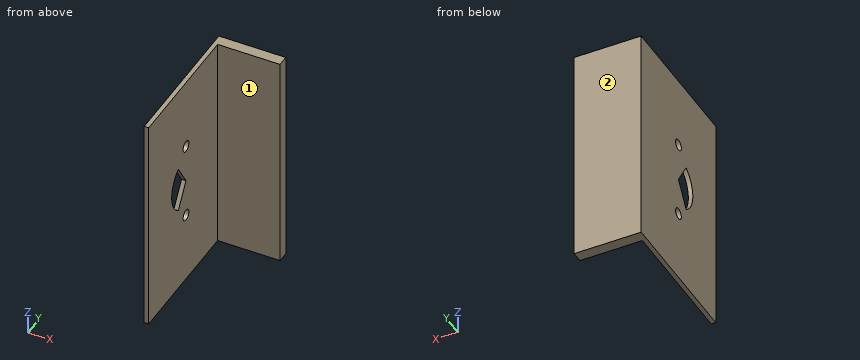
```python
from build123d import *

# Parameters (mm, degrees)
SKETCH1_W           = 100
SKETCH1_H           = 5
BOSS_EXTRUDE5_DEPTH = 2
SKETCH4_W           = 100
SKETCH4_H           = 5
BOSS_EXTRUDE6_DEPTH = 28


with BuildPart() as part:
    # Sketch1 → Boss-Extrude5 (new body)
    with BuildSketch(Plane(origin=(0, 0, 0), x_dir=(0, 0, -1), z_dir=(1, 0, 0))):
        with Locations((0, 30)):
            Rectangle(SKETCH1_W, SKETCH1_H)
        with BuildLine():
            ThreePointArc((-12.5, 0), (0, 12.5), (12.5, 0))
            Line((12.5, 0), (15, 0))
            ThreePointArc((15, 0), (17.5, 2.5), (20, 0))
            Line((20, 0), (50, 0))
            Line((50, 0), (50, 27.5))
            Line((50, 27.5), (-50, 27.5))
            Line((-50, 27.5), (-50, 0))
            Line((-50, 0), (-20, 0))
            ThreePointArc((-20, 0), (-17.5, 2.5), (-15, 0))
            Line((-15, 0), (-12.5, 0))
        make_face()
        with BuildLine():
            Line((-12.5, 0), (0, 0))
            Line((0, 0), (12.5, 0))
            ThreePointArc((12.5, 0), (0, 12.5), (-12.5, 0))
        make_face()
        with BuildLine():
            Line((-10.55739691, -6.692635541), (0, 0))
            Line((0, 0), (-12.5, 0))
            ThreePointArc((-12.5, 0), (-12.00452959, -3.484432423), (-10.55739691, -6.692635541))
        make_face()
        with BuildLine():
            Line((12.5, 0), (0, 0))
            Line((0, 0), (10.55739691, -6.692635541))
            ThreePointArc((10.55739691, -6.692635541), (12.00452959, -3.484432423), (12.5, 0))
        make_face()
        with BuildLine():
            ThreePointArc((10.55739691, -6.692635541), (0, -12.5), (-10.55739691, -6.692635541))
            ThreePointArc((-10.55739691, -6.692635541), (-12.00452959, -3.484432423), (-12.5, 0))
            Line((-12.5, 0), (-15, 0))
            ThreePointArc((-15, 0), (-17.5, -2.5), (-20, 0))
            Line((-20, 0), (-50, 0))
            Line((-50, 0), (-50, -32.5))
            Line((-50, -32.5), (50, -32.5))
            Line((50, -32.5), (50, 0))
            Line((50, 0), (20, 0))
            ThreePointArc((20, 0), (17.5, -2.5), (15, 0))
            Line((15, 0), (12.5, 0))
            ThreePointArc((12.5, 0), (12.00452959, -3.484432423), (10.55739691, -6.692635541))
        make_face()
    extrude(amount=BOSS_EXTRUDE5_DEPTH)

    # Sketch4 → Boss-Extrude6 (add)
    with BuildSketch(Plane(origin=(2, 0, 0), x_dir=(0, 0, -1), z_dir=(1, 0, 0))):
        with Locations((0, 30)):
            Rectangle(SKETCH4_W, SKETCH4_H)
    extrude(amount=BOSS_EXTRUDE6_DEPTH)


solid = part.part
```
Design review of the part built by this model. Coordinates are the model's own, in mm. Face numbers are marked on the shaded views. A direction names the side the tool comes from. Give positions to 0.01 mm unless a question says otherwise; leave off trailing zeros. Loops run counter-clockwise (first coordinate to the right, second up) from the corner with the lowest first, then second, coordinate; pieces in that order, holes last. Notation, with made-up numbers: (8.25, 18.5) -> (63.25, 18.5) arc R13 cw to (63.25, 25.5) -> close; hole circle Ø2 at (26, 66.5). An arc over 180 degrees is marked (long way). Write each question's results on one line, items separated by ' | '.
Q1. Take a section at C-C, the plane x = 26. Write out the cut boundary in (y, z), plus the area to 3 significant figures.
Reply:
outline: (27.5, -50) -> (32.5, -50) -> (32.5, 50) -> (27.5, 50) -> close | area: 500 mm²
Q2. Machinability: for the marked faces 1 and 2, which of the approach directions +Z, -Z, +X, -X, +Y, -Y give a long, thin tool a straight path to every point of the face, cutting with its end or side? Answer none if there is none.
Reply:
face 1: +Z, -Z, +X, -Y | face 2: +Z, -Z, +X, -X, +Y
Q3. Wall thickness on L1, parallel to Y at x = 1.1, z = -17.5; L2, parallel to Y at x = 28.5, z = -24; L3, parallel to X at y = 15.5, z = -41: over which ranges is each line inside the solid? List them lowest first.
Reply:
L1: y = -32.5 to -2.5, 2.5 to 32.5 | L2: y = 27.5 to 32.5 | L3: x = 0 to 2
Q4. For pin 1 Ø8 at (x, z) = (21, 30) entering from -Y; pin 2 Ø8 at (y, z) = (0, 17.5) entering from +X, all flat-tipped, find the tip position at first contact; note any pin that passes through.
Reply:
pin 1: stops at y = 27.5 | pin 2: stops at x = 2
Q5. Take a section at B-B, the plane y = 1. Write out the cut boundary in (x, z), plus the area to 3 significant figures.
Reply:
outline: (0, -50) -> (2, -50) -> (2, -19.79) -> (0, -19.79) -> close; (0, -15.21) -> (2, -15.21) -> (2, 15.21) -> (0, 15.21) -> close; (0, 19.79) -> (2, 19.79) -> (2, 50) -> (0, 50) -> close | area: 182 mm²
Q6. Take a section at D-D, the plane z = -36.5. Write out the cut boundary in (x, y), plus the area to 3 significant figures.
Reply:
outline: (0, -32.5) -> (2, -32.5) -> (2, 27.5) -> (30, 27.5) -> (30, 32.5) -> (0, 32.5) -> close | area: 270 mm²
Q7. Take a section at A-A, the plane z = 17.5. Write out the cut boundary in (x, y), plus the area to 3 significant figures.
Reply:
outline: (0, -32.5) -> (2, -32.5) -> (2, -2.5) -> (0, -2.5) -> close; (0, 2.5) -> (2, 2.5) -> (2, 27.5) -> (30, 27.5) -> (30, 32.5) -> (0, 32.5) -> close | area: 260 mm²
